```python
from build123d import *

# Parameters (mm, degrees)
ESQUISSE1_R             = 17.5
BOSS_EXTRU_1_DEPTH      = 260
ESQUISSE2_W             = 10
ESQUISSE2_H             = 5.634133163
ENL_V_MAT_EXTRU_1_DEPTH = 135
ESQUISSE3_W             = 10
ESQUISSE3_H             = 5.967992577
ENL_V_MAT_EXTRU_2_DEPTH = 43
TROU_TARAUD_M101_D      = 8.5
TROU_TARAUD_M101_DEPTH  = 46
TROU_TARAUD_M101_TIP    = 2.553657631


with BuildPart() as part:
    # Esquisse1 → Boss.-Extru.1 (new body)
    with BuildSketch(Plane.XY):
        Circle(ESQUISSE1_R)
    extrude(amount=BOSS_EXTRU_1_DEPTH)

    # Esquisse2 → Enlèv. mat.-Extru.1 (cut)
    with BuildSketch(Plane.XY.offset(260)):
        with Locations((0, 15.317066582)):
            Rectangle(ESQUISSE2_W, ESQUISSE2_H)
    extrude(amount=-ENL_V_MAT_EXTRU_1_DEPTH, mode=Mode.SUBTRACT)

    # Esquisse3 → Enlèv. mat.-Extru.2 (cut)
    with BuildSketch(Plane(origin=(0, 0, 0), x_dir=(-1, 0, 0), z_dir=(0, 0, -1))):
        with Locations((0, 15.483996289)):
            Rectangle(ESQUISSE3_W, ESQUISSE3_H)
    extrude(amount=-ENL_V_MAT_EXTRU_2_DEPTH, mode=Mode.SUBTRACT)

    # Trou taraudé M101
    with Locations(Plane.XY.offset(260)):
        with Locations((0, 0)):
            Hole(TROU_TARAUD_M101_D / 2, depth=TROU_TARAUD_M101_DEPTH)
            with Locations((0, 0, -(TROU_TARAUD_M101_DEPTH + TROU_TARAUD_M101_TIP / 2))):  # 118° drill point
                Cone(0, TROU_TARAUD_M101_D / 2, TROU_TARAUD_M101_TIP, mode=Mode.SUBTRACT)


solid = part.part
```
Can you work these out from the model? Positions are in its coordinate system, mm. A direction names the side the tool comes from. Round coordinates to 2 decimals unless told otherwise and drop trailing zeros. Loops run counter-clockwise (first coordinate to the right, second up) from the corner with the lowest first, then second, coordinate; pieces in that order, holes last. Notation, with made-up numbers: (68.5, 83) -> (83.5, 83) arc R28 ccw to (83.5, 111) -> close; hole circle Ø3 at (43.5, 35.5). An arc over 180 degrees is marked (long way). Answer in a Markdown table with one row per item.
Item 1: We'd pull the mould along X, two halves only. Please class faces 1 (the cylindrical face through (-3.794, -17.084, 128.18)), 2 (the flat face through (0, 0, 0)), 3 (the flat face through (-5, 15, 21)): released by +X, released by -X, zero draft, split by the parting line, or undercut.
Answer block:
| item | result |
|---|---|
| face 1 | split by the parting line |
| face 2 | zero draft |
| face 3 | undercut |
Item 2: Suppose I cut it at C-C, the plane x = -11. List the corners of the cut face in (y, z) for me, plus the area to 3 significant figures.
Answer block:
| item | result |
|---|---|
| outline | (-13.61, 0) -> (13.61, 0) -> (13.61, 260) -> (-13.61, 260) -> close |
| area | 7,080 mm² |
Item 3: Suppose I cut it at D-D, the plane z = 79. List the corners of the cut face in (x, y) for me.
Answer block:
| item | result |
|---|---|
| outline | circle Ø35 at (0, 0) |
Item 4: If I drill on probe 1 along Y at (x, z) = (0, 238.5); probe 2 along X at (y, z) = (0, 231.5); probe 3 along Z at (x, y) = (0.5, 13), over which ranges is the centre line in solid material (lowest first)?
Answer block:
| item | result |
|---|---|
| probe 1 | -17.5 to -4.25, 4.25 to 12.5 |
| probe 2 | -17.5 to -4.25, 4.25 to 17.5 |
| probe 3 | 43 to 125 |
Item 5: Suppose I cut it at B-B, the plane z = 178. List the corners of the cut face in (x, y) for me.
Answer block:
| item | result |
|---|---|
| outline | (-5, 12.5) -> (-5, 16.77) arc R17.5 ccw (long way) to (5, 16.77) -> (5, 12.5) -> close |
Item 6: Suppose I cut it at A-A, the plane z = 230.5. List the corners of the cut face in (x, y) for me.
Answer block:
| item | result |
|---|---|
| outline | (-5, 12.5) -> (-5, 16.77) arc R17.5 ccw (long way) to (5, 16.77) -> (5, 12.5) -> close; hole circle Ø8.5 at (0, 0) |
Item 7: Will these pins go through, and if not, where does the flat tip stop? P1, Ø5, axis at x = 1, z = 30.5, coming from the +Y side; P2, Ø12, axis at x = 12, z = 93, coming from the -Y side; P3, Ø1.3, axis at y = 15, z = 181.5, coming from the -X side.
Answer block:
| item | result |
|---|---|
| P1 | y = 12.5 |
| P2 | y = -16.44 |
| P3 | x = -10.02 |
Item 8: On a 3-axis mill with a long thin cutter (end or side, diameter ignored), from which of +Z, -Z, +X, -X, +Y, -Y can I reach the whole of each face in a straight line? I mean faces 4 (the flat face through (4, -4, 260)), 5 (the flat face through (0, 12.5, 21)), 6 (the flat face through (5, 15, 193)), 7 (the cylindrical face through (-2.285, 3.584, 236.678)). Say none if no direction works.
Answer block:
| item | result |
|---|---|
| face 4 | +Z, +X, -X, +Y, -Y |
| face 5 | -Z, +Y |
| face 6 | +Z, +Y |
| face 7 | +Z |
